Geometry check sheet. Reference: drawing and pictorial views, mm from the part's lowest x, y, z. A direction names the side the tool comes from. Round coordinates to 2 decimals unless told otherwise and drop trailing zeros. Loops run counter-clockwise (first coordinate to the right, second up) from the corner with the lowest first, then second, coordinate; pieces in that order, holes last. Notation, with made-up numbers: (-28, 20.5) - (3, 20.5) arc R14 cw to (3, 39.5) - close; hole circle Ø10 at (28.5, 38). An arc over 180 degrees is marked (long way). Put each result on its own line as item: value. Start each with the question number.
Item 1: Gauge pin test, flat ends, axial feed: pin 1 Ø5 at (y, z) = (17.5, 9) entering from +X; pin 2 Ø5 at (x, z) = (8.5, 8) entering from -Y; pin 3 Ø2 at (y, z) = (14, 9.5) entering from -X. Record the tip position at first contact, or that the pin passes through.
Item 2: Tool access check on the marked faces 1, 2 and 3. Record the directions out of +Z, -Z, +X, -X, +Y, -Y that give a thin tool (end or side, any length) a straight path to the whole face; none if there is none.
Item 3: Section check D-D, the plane x = 14.75. Record the cut outline in (y, z).
Item 4: Material ranges on line 1 along Z through (x, y) = (4.75, 11) (1 decimal); line 2 along Z through (x, y) = (18.25, 15.5); line 3 along X through (y, z) = (31.5, 5), recorded low to high.
Item 5: Section check B-B, the plane x = 9.25. Record the cut outline in (y, z), and give its area (3 significant figures).
Item 6: Section check C-C, the plane z = 1.75. Record the cut outline in (x, y).
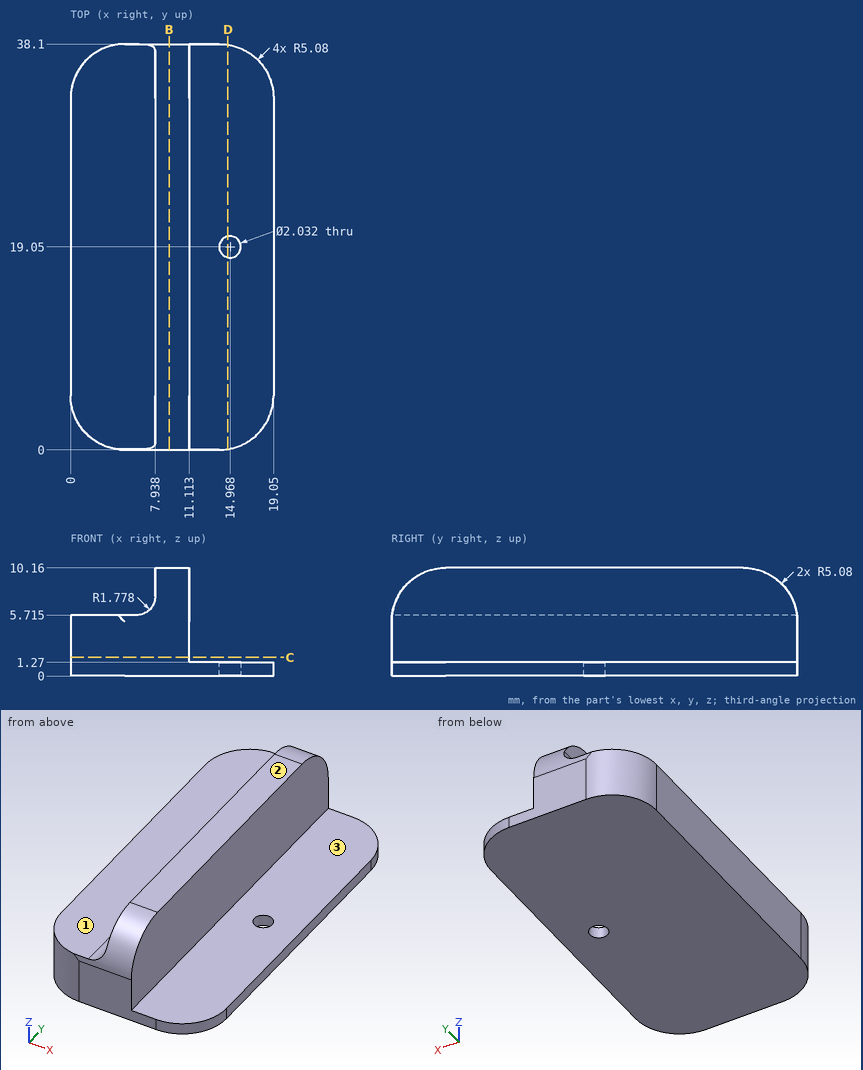
Check result:
1. pin 1: x = 11.11
1. pin 2: y = 0.02
1. pin 3: x = 7.94
2. face 1: +Z, -X, +Y, -Y
2. face 2: +Z, +X, -X, +Y, -Y
2. face 3: +Z, +X, +Y, -Y
3. outline: (0.06, 0) - (18.06, 0) - (18.06, 1.27) - (0.06, 1.27) - close; (20.04, 0) - (38.04, 0) - (38.04, 1.27) - (20.04, 1.27) - close
4. line 1: 0 to 5.7
4. line 2: 0 to 1.27
4. line 3: 0 to 11.11
5. outline: (0, 0) - (38.1, 0) - (38.1, 5.08) arc R5.08 ccw to (33.02, 10.16) - (5.08, 10.16) arc R5.08 ccw to (0, 5.08) - close
5. area: 376 mm²
6. outline: (0, 5.08) arc R5.08 ccw to (5.08, 0) - (11.11, 0) - (11.11, 38.1) - (5.08, 38.1) arc R5.08 ccw to (0, 33.02) - close
